Autodesk Inventor part; units mm, degrees
ref_plane "YZ Plane" through (0, 0, 0) normal (1, 0, 0) x (0, 1, 0)
ref_plane "XZ Plane" through (0, 0, 0) normal (0, 1, 0) x (-1, 0, 0)
ref_plane "XY Plane" through (0, 0, 0) normal (0, 0, 1) x (1, 0, 0)
sketch "Sketch1" plane through (0, 0, 0) normal (0, 1, 0) x (-1, 0, 0)
  circle A0 centre (0, 0) radius 11
  arc A1 (-6, 12.0934) -> (6, 12.0934) centre (0, 0) ccw
  line L0 (-6, 13.5) -> (-6, 113.5)
  line L1 (6, 113.5) -> (6, 13.5)
  line L2 (6, 12.0934) -> (6, 13.5)
  line L3 (-6, 13.5) -> (-6, 12.0934)
  arc A2 (6, 114.9066) -> (-6, 114.9066) centre (0, 127) ccw
  circle A3 centre (0, 127) radius 11
  line L4 (6, 113.5) -> (6, 114.9066)
  line L5 (-6, 113.5) -> (-6, 114.9066)
  circle A4 centre (0, 127) radius 4.5
  circle A5 centre (0, 0) radius 4.5
  dimension "d0" = 22
  dimension "d4" = 100
  dimension "d7" = 9
  dimension "d8" = 9
extrude "Extrusion1" add sketch "Sketch1" against normal blind 3 contours A0 | L3 L0 L5 A2 L4 L1 L2 A1 | A3
extrude "Extrusion2" add sketch "Sketch1" along normal blind 6 contours A0 | L3 L0 L5 A2 L4 L1 L2 A1 | A3
sketch "Sketch2" plane through (0, -3, 0) normal (0, -1, 0) x (1, 0, 0)
  arc A0 (-6, 12.0934) -> (6, 12.0934) centre (0, 0) ccw
  line L0 (6, 12.0934) -> (6, 114.9066)
  arc A1 (6, 114.9066) -> (-6, 114.9066) centre (0, 127) ccw
  line L1 (-6, 114.9066) -> (-6, 12.0934)
  circle A2 centre (0, 0) radius 4.5
  circle A3 centre (0, 127) radius 4.5
extrude "Extrusion3" add sketch "Sketch2" along normal blind 1
sketch "Sketch4" plane through (0, 6, 0) normal (0, 1, 0) x (1, 0, 0)
  line L0 (-6, -12.0934) -> (-6, -114.9066)
  line L1 (-6, -63.5) -> (6, -63.5)
  line L2 (6, -114.9066) -> (6, -12.0934)
  circle A0 centre (0, -63.5) radius 1.45
  point P0 (0, 0)
  dimension "d17" = 2.9
extrude "Extrusion5" cut sketch "Sketch4" against normal up to surface (10 mm away)
sketch "Sketch5" plane through (0, 6, 0) normal (0, 1, 0) x (1, 0, 0)
  arc A0 (6, -12.0934) -> (-6, -12.0934) centre (0, 0) ccw
  arc A1 (44.1065, -24.2547) -> (42.2109, 0.6996) centre (38.1065, -12.1613) ccw
  arc A2 (34.002, -152.0223) -> (44.1065, -127.0679) centre (38.1065, -139.1613) ccw
  circle A3 centre (38.1065, -139.1613) radius 4.5
  circle A4 centre (38.1065, -12.1613) radius 4.5
  arc A5 (-6, -114.9066) -> (6, -114.9066) centre (0, -127) ccw
  line L0 (44.1065, -105.6324) -> (44.1065, -127.0679)
  line L1 (32.1065, -105.6324) -> (32.1065, -123.0757)
  line L2 (44.1065, -105.6324) -> (44.1065, -24.2547)
  line L3 (32.1065, -105.6324) -> (32.1065, -24.2547)
  line L4 (-4.1044, -139.8609) -> (35.9659, -152.649)
  line L5 (6, -114.744) -> (32.1065, -123.0757)
  line L6 (6, -114.9066) -> (6, -12.0934)
  line L7 (6, -16.0857) -> (34.002, -25.0223)
  line L8 (4.1044, 12.8609) -> (42.2109, 0.6996)
  point P0 (32.1065, -24.4173)
extrude "Extrusion6" add sketch "Sketch5" against normal up to surface (10 mm away) contours A0 L8 A1 L2 L0 A2 L4 A5 L6 L5 L1 L3 L7
sketch "Sketch6" plane through (0, 6, 0) normal (0, 1, 0) x (1, 0, 0)
  circle A0 centre (0, -63.5) radius 1.45
  point P0 (0, 0)
extrude "Extrusion7" add sketch "Sketch6" against normal up to surface (10 mm away)
properties part number "damping_system_connector"
Here's how the part is built. I have some questions about the finished solid (model axes, mm). A direction names the side the tool comes from. Give positions to 0.01 mm unless a question says otherwise; leave off trailing zeros. Order: outer loops, then holes, each group sorted by start corner. A loop starts at its lowest first (then second) coordinate and runs counter-clockwise, first axis right, second up. Notation, with made-up numbers: (50, 3) -> (63, 3) arc R25 ccw to (63, 30) -> close; hole circle Ø8 at (-13, 62). An arc over 180 degrees is marked (long way). One line per item, written item: value. Start each with the question number.
1. Will these pins go through, and if not, where does the flat tip stop? pin 1 Ø0.8 at (y, z) = (-3.5, 79.5) entering from +X; pin 2 Ø1.5 at (x, y) = (11.5, 4.5) entering from -Z; pin 3 Ø3 at (x, y) = (35, -1.5) entering from -Z; pin 4 Ø7 at (x, z) = (0, 0) entering from -Y.
2. For faces 4 (the face through (22.891, 1.07, -6.865)), 5 (the face through (18.871, 1.07, 20.193)), 6 (the face through (44.106, 1, 76)), which set-ups out of +Z, -Z, +X, -X, +Y, -Y let a thin tool reach every point of the face, with its end or its side?
3. We'd pull the mould along X, two halves only. Please class faces 1 (the face through (-6, 1, 64)), 2 (the face through (51.583, 1.07, 11.362)), 3 (the face through (18.87, 1.07, 118.85)): released by +X, released by -X, zero draft, split by the parting line, or undercut.
4. Imagine slicing it at B-B, the plane x = 17.5. List the corners of the cut face in (y, z) for me, plus the area to 3 significant figures.
5. Imagine slicing it at C-C, the plane y = 1.5. List the corners of the cut face in (x, z) for me.
6. I need wall thicknesses on probe 1 along X at (y, z) = (-0.75, 109.5); probe 2 along Z at (x, y) = (0, -2.25); probe 3 along X at (y, z) = (-1.8, 127). Which ranges of each line are inside material? Lowest first, please. Write a range as from..to.
7. Imagine slicing it at A-A, the plane x = -2. List the corners of the cut face in (y, z) for me, plus the area to 3 significant figures.
Values follow:
1. pin 1: stops at x = 44.11
1. pin 2: stops at z = -10.74
1. pin 3: stops at z = -3.48
1. pin 4: passes through
2. face 4: -Z, +X, +Y, -Y
2. face 5: +Y, -Y
2. face 6: +X, +Y, -Y
3. face 1: released by -X
3. face 2: released by +X
3. face 3: undercut
4. outline: (-4, -8.59) -> (6, -8.59) -> (6, 19.76) -> (-4, 19.76) -> close; (-4, 118.41) -> (6, 118.41) -> (6, 146.76) -> (-4, 146.76) -> close
4. area: 567 mm2
5. outline: (-6, 12.09) arc R13.5 ccw to (4.1, -12.86) -> (42.21, -0.7) arc R13.5 ccw to (44.11, 24.25) -> (44.11, 127.07) arc R13.5 ccw to (34, 152.02) -> (-4.1, 139.86) arc R13.5 ccw to (-6, 114.91) -> close; hole circle Ø9 at (0, 0); hole circle Ø9 at (0, 127); hole (6, 16.09) -> (32.11, 24.42) -> (32.11, 123.08) -> (6, 114.74) -> close; hole circle Ø9 at (38.11, 12.16); hole circle Ø9 at (38.11, 139.16)
6. probe 1: x = -6..6, 32.11..44.11
6. probe 2: z = -13.5..-4.5, 4.5..122.5, 131.5..141.17
6. probe 3: x = -13.5..-4.5, 4.5..44.11
7. outline: (-4, -13.35) -> (6, -13.35) -> (6, -4.03) -> (-4, -4.03) -> close; (-4, 4.03) -> (6, 4.03) -> (6, 122.97) -> (-4, 122.97) -> close; (-4, 131.03) -> (6, 131.03) -> (6, 140.53) -> (-4, 140.53) -> close
7. area: 1,380 mm2
